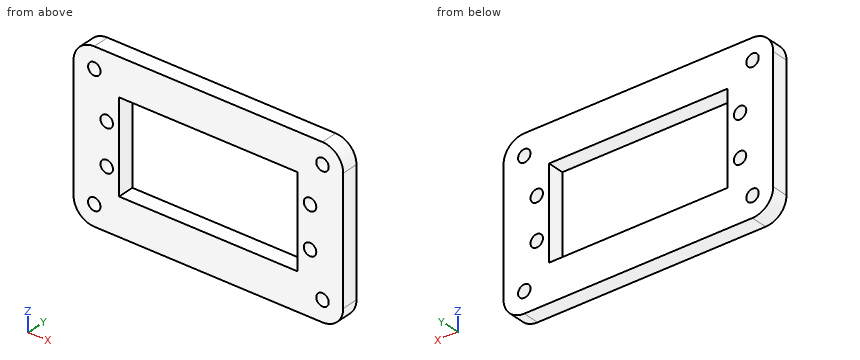
```python
from build123d import *

# Parameters (mm, degrees)
SKETCH1_W           = 65
SKETCH1_H           = 40
SKETCH1_W_2         = 43
SKETCH1_H_2         = 22
BOSS_EXTRUDE1_DEPTH = 4
SKETCH2_R           = 1.5
CUT_EXTRUDE1_DEPTH  = 39.369910086
FILLET1_R           = 5
FILLET2_R           = 5
FILLET3_R           = 5
FILLET4_R           = 5


with BuildPart() as part:
    # Sketch1 → Boss-Extrude1 (new body)
    with BuildSketch(Plane(origin=(0, 0, 0), x_dir=(1, 0, 0), z_dir=(0, 1, 0))):
        Rectangle(SKETCH1_W, SKETCH1_H)
        Rectangle(SKETCH1_W_2, SKETCH1_H_2, mode=Mode.SUBTRACT)
    extrude(amount=BOSS_EXTRUDE1_DEPTH)

    # Sketch2 → Cut-Extrude1 (cut, through all)
    with BuildSketch(Plane(origin=(0, 4, 0), x_dir=(1, 0, 0), z_dir=(0, 1, 0))):
        with Locations(Location((-24.5, 5.504503052, 0), (0, 0, 270))):
            Circle(SKETCH2_R)
        with Locations(Location((-24.5, -4.495496948, 0), (0, 0, 270))):
            Circle(SKETCH2_R)
        with Locations(Location((24.5, 5, 0), (0, 0, 270))):
            Circle(SKETCH2_R)
        with Locations(Location((24.5, -5, 0), (0, 0, 270))):
            Circle(SKETCH2_R)
        with Locations(Location((-27.5, 15, 0), (0, 0, 270))):
            Circle(SKETCH2_R)
        with Locations(Location((27.5, 15, 0), (0, 0, 270))):
            Circle(SKETCH2_R)
        with Locations(Location((27.5, -15, 0), (0, 0, 270))):
            Circle(SKETCH2_R)
        with Locations(Location((-27.5, -15, 0), (0, 0, 270))):
            Circle(SKETCH2_R)
    extrude(amount=-CUT_EXTRUDE1_DEPTH, mode=Mode.SUBTRACT)

    # Fillet1
    fillet1_edges = [part.edges().sort_by_distance(p)[0] for p in [
        (-32.5, 2, -20),
    ]]
    fillet(fillet1_edges, radius=FILLET1_R)

    # Fillet2
    fillet2_edges = [part.edges().sort_by_distance(p)[0] for p in [
        (32.5, 2, -20),
    ]]
    fillet(fillet2_edges, radius=FILLET2_R)

    # Fillet3
    fillet3_edges = [part.edges().sort_by_distance(p)[0] for p in [
        (32.5, 2, 20),
    ]]
    fillet(fillet3_edges, radius=FILLET3_R)

    # Fillet4
    fillet4_edges = [part.edges().sort_by_distance(p)[0] for p in [
        (-32.5, 2, 20),
    ]]
    fillet(fillet4_edges, radius=FILLET4_R)


solid = part.part
```
Geometry: final body of the model. Coordinates: model frame, mm. Coordinates: 2 decimals unless noted, no trailing zeros. Order: outer loops, then holes, each group sorted by start corner. A loop starts at its lowest first (then second) coordinate and runs counter-clockwise, first axis right, second up. Notation, with made-up numbers: (66, 18) -> (98, 18) arc R17 ccw to (98, 24) -> close; hole circle Ø7 at (85.5, 12). An arc over 180 degrees is marked (long way). Write each question's results on one line, items separated by ' | '. Start each with the question number.
1) Cut plane D-D, the plane x = -24.5. Output: boundary loops of the cut face in (y, z), and give its area (3 significant figures).
2) Cut plane C-C, the plane z = 9.5. Output: boundary loops of the cut face in (x, y).
3) Cut plane B-B, the plane y = 1.2. State how many separate pieces and enclosed holes the cut face has, and give its area (3 significant figures).
4) Cut plane A-A, the plane x = 0. Output: boundary loops of the cut face in (y, z).
5) Material intervals for line 1 along X through (y, z) = (1.5, 15); line 2 along X through (y, z) = (1.3, -1.5); line 3 along Z through (x, y) = (16.5, 0.2), sorted ascending.
Checks:
1) outline: (0, -20) -> (4, -20) -> (4, -7) -> (0, -7) -> close; (0, -4) -> (4, -4) -> (4, 3) -> (0, 3) -> close; (0, 6) -> (4, 6) -> (4, 20) -> (0, 20) -> close | area: 136 mm^2
2) outline: (-32.5, 0) -> (-21.5, 0) -> (-21.5, 4) -> (-32.5, 4) -> close; (21.5, 0) -> (32.5, 0) -> (32.5, 4) -> (21.5, 4) -> close
3) separate pieces: 1 | enclosed holes: 9 | area: 1,580 mm^2
4) outline: (0, -20) -> (4, -20) -> (4, -11) -> (0, -11) -> close; (0, 11) -> (4, 11) -> (4, 20) -> (0, 20) -> close
5) line 1: -32.5 to -29, -26 to 26, 29 to 32.5 | line 2: -32.5 to -21.5, 21.5 to 32.5 | line 3: -20 to -11, 11 to 20
